Input: dimensioned drawing with shaded views. Units: mm. Origin: part minimum x, y, z. A direction names the side the tool comes from. Round coordinates to 2 decimals unless told otherwise and drop trailing zeros. Loops run counter-clockwise (first coordinate to the right, second up) from the corner with the lowest first, then second, coordinate; pieces in that order, holes last.
Item 1: Pull-direction query (Y, two-part tool) for the marked faces 4, 5 and 6; classes: released by +Y, released by -Y, zero draft, split by the parting line, or undercut.
Item 2: Ray query, L1, parallel to Z at x = 3.25, y = 21; L2, parallel to Y at x = 6, z = 2.5; L3, parallel to Z at x = 3.25, y = 38.5. Return the intervals inside material, ascending.
Item 3: Access query for the marked faces 1, 2 and 3. Directions: +Z, -Z, +X, -X, +Y, -Y. A direction counts if a zero-diameter tool reaches every point of the face in a straight line with its end or side. Return the directions, or none.
Item 4: Section query B-B on z = 3.25. Return loops of the section in (x, y).
Item 5: First-contact query: P1, Ø1, axis at y = 12.5, z = 2.5, coming from the +X side; P2, Ø1.5, axis at x = 2, z = 3.5, coming from the -Y side; P3, Ø1, axis at x = 2.5, y = 16, coming from the +Z side; P4, Ø1.5, axis at y = 36.5, z = 1.5, coming from the +X side. Flat tips, straight axial feed; report the tip coordinate or a pass-through.
Item 6: Section query A-A on x = 4. Return loops of the section in (y, z), then the cut area to 3 significant figures.
Item 7: Section query D-D on y = 48. Return loops of the section in (x, z) (3 decimals), then the cut area to 3 significant figures.
Item 8: Section query C-C on y = 28.5. Return loops of the section in (x, z) (3 decimals), then the cut area to 3 significant figures.
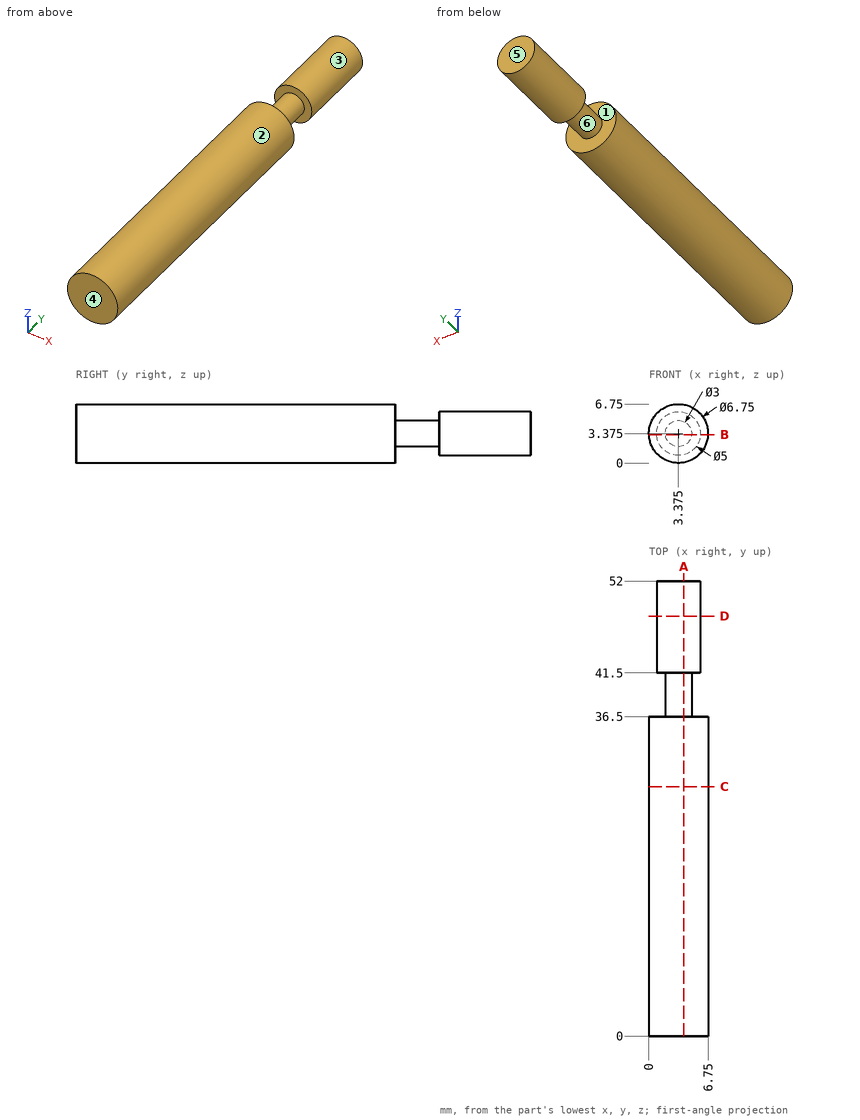
Data:
1. face 4: released by -Y
1. face 5: released by +Y
1. face 6: undercut
2. L1: z = 0 to 6.75
2. L2: y = 0 to 36.5
2. L3: z = 1.88 to 4.87
3. face 1: none
3. face 2: +Y, -Y
3. face 3: +Y
4. outline: (0, 0) - (6.75, 0) - (6.75, 36.5) - (4.87, 36.5) - (4.87, 41.5) - (5.87, 41.5) - (5.87, 52) - (0.88, 52) - (0.88, 41.5) - (1.88, 41.5) - (1.88, 36.5) - (0, 36.5) - close
5. P1: stops at x = 6.73
5. P2: stops at y = 0
5. P3: stops at z = 6.73
5. P4: stops at x = 6.56
6. outline: (0, 0.06) - (36.5, 0.06) - (36.5, 2.01) - (41.5, 2.01) - (41.5, 0.95) - (52, 0.95) - (52, 5.8) - (41.5, 5.8) - (41.5, 4.74) - (36.5, 4.74) - (36.5, 6.69) - (0, 6.69) - close
6. area: 307 mm2
7. outline: circle Ø5 at (3.375, 3.375)
7. area: 19.6 mm2
8. outline: circle Ø6.75 at (3.375, 3.375)
8. area: 35.8 mm2
